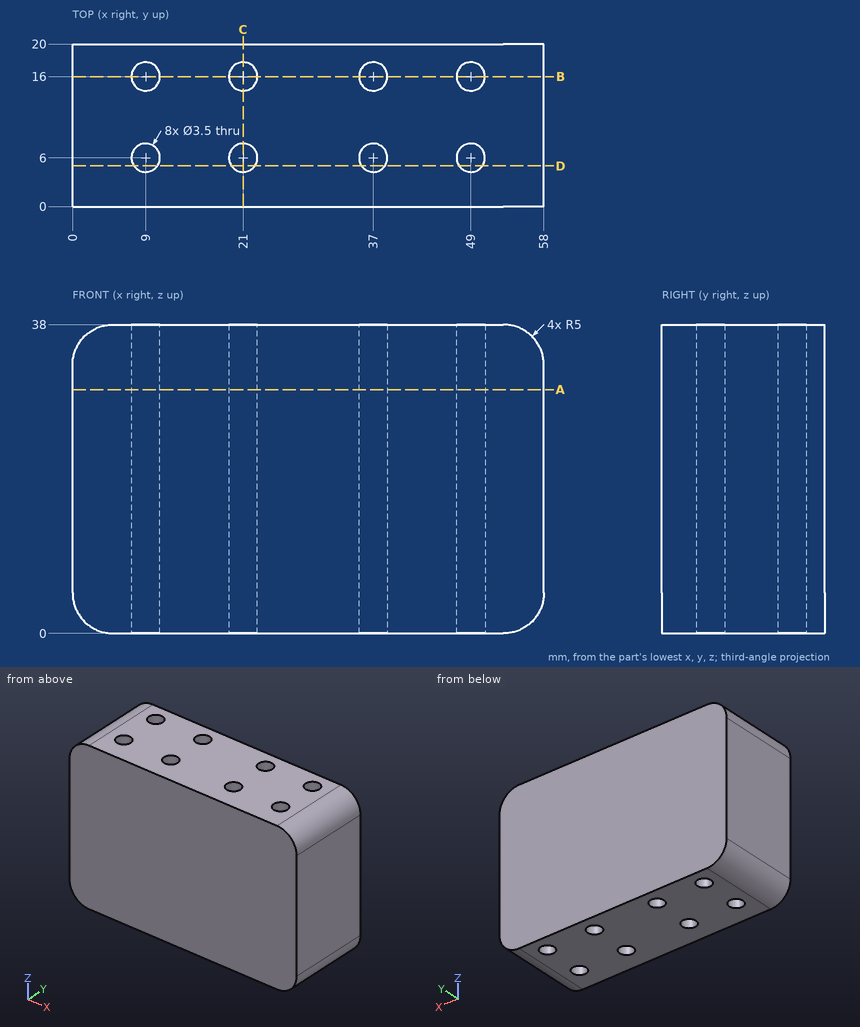
Answer from the drawing. Dimensions are ordinates in mm from the lowest x, y and z of the part. Round coordinates to 2 decimals unless told otherwise and drop trailing zeros. Loops run counter-clockwise (first coordinate to the right, second up) from the corner with the lowest first, then second, coordinate; pieces in that order, holes last.
Q1. Section B-B on y = 16 is taken. Write down the section's boundary in (x, z).
Q2. Section A-A on z = 30 is taken. Give the number of separate pieces and of enclosed holes in the cut face, and give its area (3 significant figures).
Q3. Consider probe 1 along Y at (x, z) = (49, 21); probe 2 along X at (y, z) = (17, 21); probe 3 along Y at (x, z) = (47.5, 31). Determine where each line is inside the solid, lowest interval first.
Q4. Section C-C on x = 21 is taken. Write down the section's boundary in (y, z), and give its area (3 significant figures).
Q5. Section D-D on y = 5 is taken. Write down the section's boundary in (x, z), and give its area (3 significant figures).
Q6. This flat-tipped pin is pushed along its axis until it touches: pin 1 (12 mm diameter, centred on y = 13.5, z = 10, fed in from -X). Where does it stop, or does it pass through?
Output:
1. outline: (0, 5) arc R5 ccw to (5, 0) - (7.25, 0) - (7.25, 38) - (5, 38) arc R5 ccw to (0, 33) - close; (10.75, 0) - (19.25, 0) - (19.25, 38) - (10.75, 38) - close; (22.75, 0) - (35.25, 0) - (35.25, 38) - (22.75, 38) - close; (38.75, 0) - (47.25, 0) - (47.25, 38) - (38.75, 38) - close; (50.75, 0) - (53, 0) arc R5 ccw to (58, 5) - (58, 33) arc R5 ccw to (53, 38) - (50.75, 38) - close
2. separate pieces: 1
2. enclosed holes: 8
2. area: 1,080 mm2
3. probe 1: y = 0 to 4.25, 7.75 to 14.25, 17.75 to 20
3. probe 2: x = 0 to 7.56, 10.44 to 19.56, 22.44 to 35.56, 38.44 to 47.56, 50.44 to 58
3. probe 3: y = 0 to 5.1, 6.9 to 15.1, 16.9 to 20
4. outline: (0, 0) - (4.25, 0) - (4.25, 38) - (0, 38) - close; (7.75, 0) - (14.25, 0) - (14.25, 38) - (7.75, 38) - close; (17.75, 0) - (20, 0) - (20, 38) - (17.75, 38) - close
4. area: 494 mm2
5. outline: (0, 5) arc R5 ccw to (5, 0) - (7.56, 0) - (7.56, 38) - (5, 38) arc R5 ccw to (0, 33) - close; (10.44, 0) - (19.56, 0) - (19.56, 38) - (10.44, 38) - close; (22.44, 0) - (35.56, 0) - (35.56, 38) - (22.44, 38) - close; (38.44, 0) - (47.56, 0) - (47.56, 38) - (38.44, 38) - close; (50.44, 0) - (53, 0) arc R5 ccw to (58, 5) - (58, 33) arc R5 ccw to (53, 38) - (50.44, 38) - close
5. area: 1,750 mm2
6. pin 1: stops at x = 0
